Here's how the part is built. I have some questions about the finished solid (model axes, mm). Face numbers are marked on the shaded views. A direction names the side the tool comes from. Round coordinates to 2 decimals unless told otherwise and drop trailing zeros. Order: outer loops, then holes, each group sorted by start corner. A loop starts at its lowest first (then second) coordinate and runs counter-clockwise, first axis right, second up.
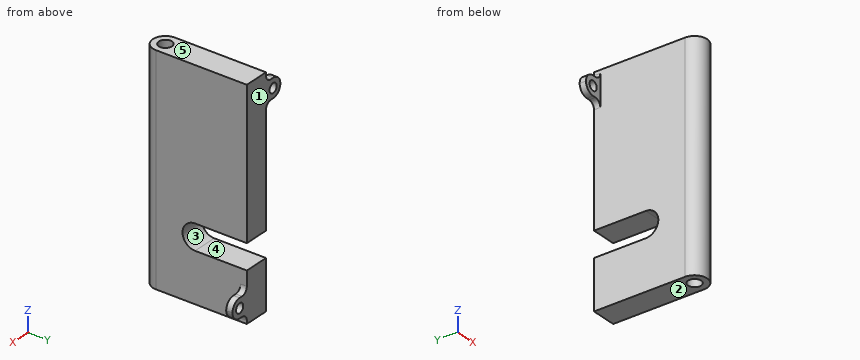
Autodesk Inventor part; units mm, degrees
ref_plane "YZ Plane" through (0, 0, 0) normal (1, 0, 0) x (0, 1, 0)
ref_plane "XZ Plane" through (0, 0, 0) normal (0, 1, 0) x (-1, 0, 0)
ref_plane "XY Plane" through (0, 0, 0) normal (0, 0, 1) x (1, 0, 0)
sketch "Sketch7" plane through (0, 0, 0) normal (0, 0, 1) x (1, 0, 0)
  circle A0 centre (0, 0) radius 4
  arc A1 (-8, 0) -> (8, 0) centre (0, 0) ccw
  line L0 (-8, 54) -> (-20, 54)
  line L1 (-20, 54) -> (-20, 58)
  line L2 (-20, 58) -> (0, 58)
  line L3 (0, 58) -> (20, 58)
  line L4 (20, 58) -> (20, 54)
  line L5 (20, 54) -> (8, 54)
  line L6 (-8, 0) -> (-8, 54)
  line L7 (8, 0) -> (8, 54)
  dimension "d34" = 4
  dimension "d35" = 58
  dimension "d36" = 8
  dimension "d37" = 4
  dimension "d38" = 12
extrude "Extrusion6" add sketch "Sketch7" along normal blind 140
sketch "Sketch8" plane through (-20, 54, 0) normal (0, -1, 0) x (1, 0, 0)
  line L0 (12, 140) -> (0, 140)
  line L1 (0, 0) -> (0, 140)
  line L2 (0, 0) -> (12, 0)
  line L3 (12, 0) -> (12, 140)
  line L4 (40, 140) -> (28, 140)
  line L5 (28, 0) -> (28, 140)
  line L6 (28, 0) -> (40, 0)
  line L7 (40, 0) -> (40, 140)
  line L8 (0, 134) -> (12, 134)
  line L9 (12, 134) -> (12, 122)
  line L10 (12, 122) -> (0, 122)
  line L11 (0, 122) -> (0, 134)
  line L12 (28, 6) -> (40, 6)
  line L13 (40, 6) -> (40, 18)
  line L14 (40, 18) -> (28, 18)
  line L15 (28, 18) -> (28, 6)
  point P0 (20, 0)
  dimension "d41" = 12
  dimension "d42" = 6
  dimension "d43" = 6
extrude "Extrusion7" cut sketch "Sketch8" against normal blind 140 contours L3 L8 L1 L0 | L3 L2 L1 L10 | L7 L14 L5 L4 | L7 L6 L5 L12
fillet "Fillet1" radius 6 4 edges at (20, 56, 6) (20, 56, 18) (-20, 56, 134) (-20, 56, 122)
fillet "Fillet1" radius 4 4 edges at (-8, 56, 134) (-8, 56, 122) (8, 56, 6) (8, 56, 18)
sketch "Sketch9" plane through (-14, 54, 122) normal (0, -1, 0) x (1, 0, 0)
  arc A0 (0, 12) -> (0, 0) centre (0, 6) ccw
  arc A1 (28, -116) -> (28, -104) centre (28, -110) ccw
  line L0 (28, -104) -> (26, -104)
  arc A2 (22, -100) -> (26, -104) centre (26, -100) ccw
  line L1 (22, -120) -> (22, -100)
  arc A3 (26, -116) -> (22, -120) centre (26, -120) ccw
  line L2 (26, -116) -> (28, -116)
  point P0 (14, -122)
hole "Hole2" at (14, 54, 12) at (-14, 54, 128) direction (0, 1, 0) diameter 6 depth 8 tip angle 118
sketch "Sketch10" plane through (0, 0, 140) normal (0, 0, 1) x (1, 0, 0)
  arc A0 (-8, 0) -> (8, 0) centre (0, 0) ccw
hole "Hole3" at (0, 0, 140) direction (0, 0, -1) diameter 8.376 depth 20 tip angle 118
sketch "Sketch11" plane through (0, 0, 0) normal (0, 0, -1) x (-1, 0, 0)
  arc A0 (-8, 0) -> (8, 0) centre (0, 0) ccw
hole "Hole4" at (0, 0, 0) direction (0, 0, 1) diameter 8.376 depth 20 tip angle 118
ref_plane "Work Plane3" through (0, 0, 140) normal (1, 0, 0) x (0, 0, -1)
sketch "Sketch12" plane through (-8, 0, 0) normal (-1, 0, 0) x (0, 0, 1)
  line L0 (0, 58) -> (118, 58)
  arc A0 (31.2994, 25) -> (47.2994, 25) centre (39.2994, 25) ccw
  line L1 (47.2994, 58) -> (47.2994, 25)
  line L2 (31.2994, 58) -> (31.2994, 25)
  circle A1 centre (39.2994, 25) radius 8
  line L3 (31.2994, 25) -> (31.2994, 58)
  line L4 (47.2994, 25) -> (47.2994, 58)
extrude "Extrusion8" cut sketch "Sketch12" against normal through all
properties part number "Pusher.Holder2" material "Aluminum-6061"
1) I need wall thicknesses on line 1 (X direction, y = 56, z = 128); line 2 (Z direction, x = -5, y = 31.5); line 3 (X direction, y = 56.9, z = 12). Which ranges of each line are inside material? Lowest first, please.
2) If we section it at D-D (x = 6): Write out the boundary of the cut face in (y, z), plus the area to 3 significant figures.
3) If we section it at B-B (x = 0): Write out the boundary of the cut face in (y, z), plus the area to 3 significant figures.
4) For the marked faces 4 and 5, which set-ups out of +Z, -Z, +X, -X, +Y, -Y let a thin tool reach every point of the face, with its end or its side?
5) We'd pull the mould along Z, two halves only. Please class the marked faces 1, 2 and 3: +Z half, -Z half, draft (parallel to the pull), parting line (faces both ways), or undercut.
6) If we section it at A-A (y = 49.5): Write out the boundary of the cut face in (x, z).
7) I'm going to push flat-ended pins straight in: pin 1 (2 mm diameter, centred on x = -12.5, y = 56, fed in from -Z); pin 2 (1 mm diameter, centred on y = 48, z = 70.5, fed in from -X); pin 3 (0.6 mm diameter, centred on x = -13, y = 55, fed in from +Z). Where does each tip first touch, or does it pass through?
8) If we section it at C-C (z = 61.5): Write out the boundary of the cut face in (x, y).
Solutions:
1. line 1: x = -20 to -17, -11 to 8
1. line 2: z = 0 to 31.3, 47.3 to 140
1. line 3: x = -8 to 11, 17 to 20
2. outline: (-5.29, 0) - (58, 0) - (58, 31.3) - (25, 31.3) arc R8 cw to (25, 47.3) - (58, 47.3) - (58, 140) - (-5.29, 140) - close
2. area: 8,230 mm2
3. outline: (-8, 0) - (-4.19, 0) - (-4.19, 20) - (-4, 20.11) - (-4, 119.89) - (-4.19, 120) - (-4.19, 140) - (-8, 140) - close; (4, 20.11) - (4.19, 20) - (4.19, 0) - (58, 0) - (58, 31.3) - (25, 31.3) arc R8 cw to (25, 47.3) - (58, 47.3) - (58, 140) - (4.19, 140) - (4.19, 120) - (4, 119.89) - close
3. area: 7,480 mm2
4. face 4: +X, -X, +Y
4. face 5: +Z, +X, -X, +Y, -Y
5. face 1: draft
5. face 2: -Z half
5. face 3: undercut
6. outline: (-8, 0) - (8, 0) - (8, 31.3) - (-8, 31.3) - close; (-8, 47.3) - (8, 47.3) - (8, 140) - (-8, 140) - close
7. pin 1: stops at z = 121.97
7. pin 2: stops at x = -8
7. pin 3: stops at z = 134
8. outline: (-8, 0) arc R8 ccw to (8, 0) - (8, 58) - (-8, 58) - close; hole circle Ø8 at (0, 0)
